from build123d import *

# Parameters (mm, degrees)
BASE_FLANGE1_DEPTH = 63.5
SKETCH6_R          = 2.38125
CUT_EXTRUDE1_DEPTH = 25.4
SKETCH7_R          = 3.430168193
CUT_EXTRUDE2_DEPTH = 25.4


# Sheet-metal steps are written as plain solids
with BuildPart() as part:
    # Sketch1 → Base-Flange1 (new body)
    with BuildSketch(Plane(origin=(0, 0, 0), x_dir=(0, 0, -1), z_dir=(1, 0, 0))):
        with BuildLine():
            Line((-25.4, 0), (-5.83184, 0))
            ThreePointArc((-5.83184, 0), (-1.708106389, 1.708106389), (0, 5.83184))
            Line((0, 5.83184), (0, 101.6))
            Line((0, 101.6), (-2.65684, 101.6))
            Line((-2.65684, 101.6), (-2.65684, 5.83184))
            ThreePointArc((-2.65684, 5.83184), (-3.58677597, 3.58677597), (-5.83184, 2.65684))
            Line((-5.83184, 2.65684), (-25.4, 2.65684))
            Line((-25.4, 2.65684), (-25.4, 0))
        make_face()
    extrude(amount=BASE_FLANGE1_DEPTH)

    # Sketch6 → Cut-Extrude1 (cut)
    with BuildSketch(Plane(origin=(0, 2.65684, 0), x_dir=(1, 0, 0), z_dir=(0, 1, 0))):
        with Locations(Location((6.35, -10.27684, 0), (0, 0, 270))):
            Circle(SKETCH6_R)
        with Locations(Location((57.15, -10.27684, 0), (0, 0, 270))):
            Circle(SKETCH6_R)
    extrude(amount=-CUT_EXTRUDE1_DEPTH, mode=Mode.SUBTRACT)

    # Sketch7 → Cut-Extrude2 (cut)
    with BuildSketch(Plane.XY.offset(2.65684)):
        with Locations((57.15, 49.268253676)):
            Circle(SKETCH7_R)
        with Locations((57.15, 74.668253676)):
            Circle(SKETCH7_R)
        with Locations((57.15, 23.868253676)):
            Circle(SKETCH7_R)
    extrude(amount=-CUT_EXTRUDE2_DEPTH, mode=Mode.SUBTRACT)


solid = part.part
Could you check a few things on this model? Use its own coordinates, in mm. A direction names the side the tool comes from. Give positions to 0.01 mm unless a question says otherwise; leave off trailing zeros. Write each loop counter-clockwise with the first axis right and the second up, starting at its lowest first coordinate (ties: lowest second). Pieces come first, ordered by that corner, then holes. Notation, with made-up numbers: (55, 56.5) -> (81, 56.5) arc R19 ccw to (81, 72.5) -> close; hole circle Ø7 at (80.25, 37). An arc over 180 degrees is marked (long way). Answer as CSV lines item,"result". Start each with the question number.
(1) If we section it at A-A, the plane x = 6.35: Write out the boundary of the cut face in (y, z) (3 decimals), and give its area (3 significant figures).
(2) Which directions (+Z, -Z, +X, -X, +Y, -Y) give clear straight access to the entire face, cutting with the end or side of a thin tool? Please do faces 1 (the face through (31.306, 1.663, 1.754)), 2 (the face through (31, 54, 2.657)).
(3) If we section it at B-B, the plane x = 57.15: Write out the boundary of the cut face in (y, z) (3 decimals).
(4) Please list where these lines run through material, in increasing order: line 1 (Y direction, x = 57.15, z = 1.55); line 2 (Y direction, x = 5, z = 8).
(5) If we section it at C-C, the plane y = 25.5: Write out the boundary of the cut face in (x, z), and give its area (3 significant figures).
(6) If we mould it in two halves opening along X, with no side actions, what happens to faces 3 (the face through (59.51, 1.35, 9.97)), 4 (the face through (0, 40, 2)), 5 (the face through (31, 2.657, 15))? For each: +X half, -X half, draft (parallel to the pull), parting line (faces both ways), or undercut.
(7) If we section it at D-D, the plane z = 9.5: Write out the boundary of the cut face in (x, y).
(8) I'm going to push flat-ended pins straight in: pin 1 Ø12 at (y, z) = (88, 11) entering from -X; pin 2 Ø10 at (x, z) = (36.5, 16.5) entering from +Y; pin 3 Ø19 at (x, y) = (19, 42.5) entering from +Z. Where does each tip first touch, or does it pass through?
Answer list:
1,outline,"(0, 5.832) arc R5.832 ccw to (5.832, 0) -> (101.6, 0) -> (101.6, 2.657) -> (5.832, 2.657) arc R3.175 cw to (2.657, 5.832) -> (2.657, 7.896) -> (0, 7.896) -> close; (0, 12.658) -> (2.657, 12.658) -> (2.657, 25.4) -> (0, 25.4) -> close"
1,area,"313 mm^2"
2,face 1,"-Z, +X, -X, -Y"
2,face 2,"+Z, +X, -X, +Y"
3,outline,"(0, 5.832) arc R5.832 ccw to (5.832, 0) -> (20.438, 0) -> (20.438, 2.657) -> (5.832, 2.657) arc R3.175 cw to (2.657, 5.832) -> (2.657, 7.896) -> (0, 7.896) -> close; (0, 12.658) -> (2.657, 12.658) -> (2.657, 25.4) -> (0, 25.4) -> close; (27.298, 0) -> (45.838, 0) -> (45.838, 2.657) -> (27.298, 2.657) -> close; (52.698, 0) -> (71.238, 0) -> (71.238, 2.657) -> (52.698, 2.657) -> close; (78.098, 0) -> (101.6, 0) -> (101.6, 2.657) -> (78.098, 2.657) -> close"
4,line 1,"1.87 to 20.44, 27.3 to 45.84, 52.7 to 71.24, 78.1 to 101.6"
4,line 2,"0 to 2.66"
5,outline,"(0, 0) -> (54.13, 0) -> (54.13, 2.66) -> (0, 2.66) -> close; (60.17, 0) -> (63.5, 0) -> (63.5, 2.66) -> (60.17, 2.66) -> close"
5,area,"153 mm^2"
6,face 3,"undercut"
6,face 4,"-X half"
6,face 5,"draft"
7,outline,"(0, 0) -> (4.1, 0) -> (4.1, 2.66) -> (0, 2.66) -> close; (8.6, 0) -> (54.9, 0) -> (54.9, 2.66) -> (8.6, 2.66) -> close; (59.4, 0) -> (63.5, 0) -> (63.5, 2.66) -> (59.4, 2.66) -> close"
8,pin 1,"through"
8,pin 2,"y = 2.66"
8,pin 3,"z = 2.66"
